Source: CAD feature listing. Evaluate the final solid. Frame: model axes, mm. Face numbers are marked on the shaded views. A direction names the side the tool comes from. Round coordinates to 2 decimals unless told otherwise and drop trailing zeros. Write each loop counter-clockwise with the first axis right and the second up, starting at its lowest first coordinate (ties: lowest second). Pieces come first, ordered by that corner, then holes. Notation, with made-up numbers: (46.25, 38) -> (104.25, 38) arc R13 cw to (104.25, 63) -> close; hole circle Ø8 at (25, 71.25). An arc over 180 degrees is marked (long way). Put each result on its own line as item: value.
```python
from build123d import *

# Parameters (mm, degrees)
F0_R     = 7.5
F0_R_2   = 10
F1_DEPTH = 10


with BuildPart() as f1:
    # F0 (on Front) → F1 (new body)
    with BuildSketch(Plane.XZ):
        with BuildLine():
            ThreePointArc((-15, 75), (0, 60), (15, 75))
            ThreePointArc((15, 75), (0, 90), (-15, 75))
        make_face()
        with Locations((0, 75)):
            Circle(F0_R, mode=Mode.SUBTRACT)
        with BuildLine():
            Line((15, 35.980762), (15, 75))
            ThreePointArc((15, 75), (0, 60), (-15, 75))
            Line((-15, 75), (-15, 0))
            ThreePointArc((-15, 0), (0, 15), (15, 0))
            ThreePointArc((15, 0), (12.990381, -7.5), (7.5, -12.990381))
            Line((7.5, -12.990381), (85.442286, 32.009619))
            ThreePointArc((85.442286, 32.009619), (64.951905, 37.5), (70.442286, 57.990381))
            Line((70.442286, 57.990381), (23.660254, 30.980762))
            ThreePointArc((23.660254, 30.980762), (18.803432, 32.568499), (15, 35.980762))
        make_face()
        with BuildLine():
            ThreePointArc((15, 0), (0, 15), (-15, 0))
            ThreePointArc((-15, 0), (-7.5, -12.990381), (7.5, -12.990381))
            ThreePointArc((7.5, -12.990381), (12.990381, -7.5), (15, 0))
        make_face()
        Circle(F0_R_2, mode=Mode.SUBTRACT)
        with BuildLine():
            ThreePointArc((92.942286, 45), (85.442286, 57.990381), (70.442286, 57.990381))
            ThreePointArc((70.442286, 57.990381), (64.951905, 37.5), (85.442286, 32.009619))
            ThreePointArc((85.442286, 32.009619), (90.932667, 37.5), (92.942286, 45))
        make_face()
        with Locations((77.942286, 45)):
            Circle(F0_R, mode=Mode.SUBTRACT)
    extrude(amount=F1_DEPTH)


solid = f1.part
```
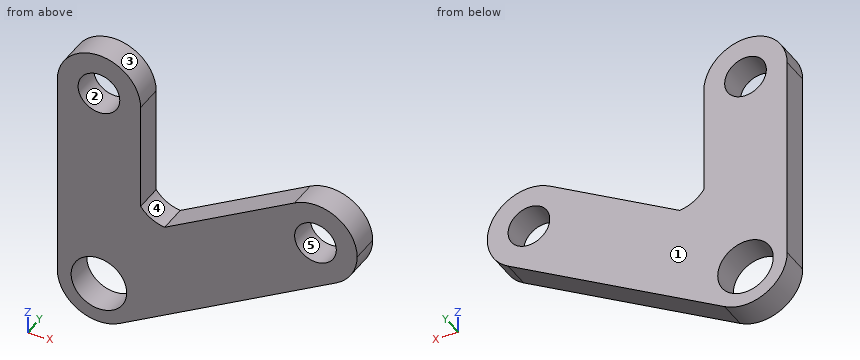
Q1. Draft query along X for the marked faces 1, 2 and 3. Return one class per face: +X half, -X half, draft (parallel to the pull), parting line (faces both ways), or undercut.
Ans:
face 1: draft
face 2: undercut
face 3: parting line
Q2. Reachability of the marked faces 4 and 5 from +Z, -Z, +X, -X, +Y, -Y: full face, straight path, thin tool, end or side. Return the list, or none.
Ans:
face 4: +Z, +Y, -Y
face 5: +Y, -Y
Q3. Cut plane A-A on x = 0. Output: boundary loops of the cut face in (y, z), and give its area (3 significant figures).
Ans:
outline: (-10, -15) -> (0, -15) -> (0, -10) -> (-10, -10) -> close; (-10, 10) -> (0, 10) -> (0, 67.5) -> (-10, 67.5) -> close; (-10, 82.5) -> (0, 82.5) -> (0, 90) -> (-10, 90) -> close
area: 700 mm^2
Q4. Material intervals for line 1 (Z direction, x = 0, y = -6.25); line 2 (X direction, y = -4, z = 48.5); line 3 (Z direction, x = -1, y = -4.5), sorted ascending. Write a range as [from, to].
Ans:
line 1: z = [-15, -10], [10, 67.5], [82.5, 90]
line 2: x = [-15, 15], [54, 71.31], [84.58, 92.53]
line 3: z = [-14.97, -9.95], [9.95, 67.57], [82.43, 89.97]
Q5. Cut plane B-B on y = -3. Output: boundary loops of the cut face in (x, z), and give its area (3 significant figures).
Ans:
outline: (-15, 0) arc R15 ccw to (7.5, -12.99) -> (85.44, 32.01) arc R15 ccw to (70.44, 57.99) -> (23.66, 30.98) arc R12.39 cw to (15, 35.98) -> (15, 75) arc R15 ccw to (-15, 75) -> close; hole circle Ø20 at (0, 0); hole circle Ø15 at (0, 75); hole circle Ø15 at (77.94, 45)
area: 4,870 mm^2
Q6. Cut plane C-C on z = 46.5. Output: boundary loops of the cut face in (x, y).
Ans:
outline: (-15, -10) -> (15, -10) -> (15, 0) -> (-15, 0) -> close; (50.54, -10) -> (70.59, -10) -> (70.59, 0) -> (50.54, 0) -> close; (85.29, -10) -> (92.87, -10) -> (92.87, 0) -> (85.29, 0) -> close
Q7. Cut plane D-D on x = 76.5. Output: boundary loops of the cut face in (y, z).
Ans:
outline: (-10, 26.85) -> (0, 26.85) -> (0, 37.64) -> (-10, 37.64) -> close; (-10, 52.36) -> (0, 52.36) -> (0, 59.93) -> (-10, 59.93) -> close
Q8. Pin query (flat end, axial travel): pin 1 (4 mm diameter, centred on y = -2.5, z = 41.5, fed in from +X); pin 2 (23 mm diameter, centred on x = 0, z = 0, fed in from +Y); pin 3 (4 mm diameter, centred on y = -2.5, z = 18.5, fed in from +X). Return the tip coordinate at first contact, or that it passes through.
Ans:
pin 1: stops at x = 92.87
pin 2: stops at y = 0
pin 3: stops at x = 65.51
